from build123d import *

# Parameters (mm, degrees)
SKETCH1_W            = 96
SKETCH1_H            = 11.5
BOSS_EXTRUDE1_DEPTH  = 1
BOSS_EXTRUDE2_DEPTH  = 96
SKETCH3_W            = 100.030166713
SKETCH3_H            = 53.267661774
CUT_EXTRUDE1_DEPTH   = 96
SKETCH4_W            = 73
SKETCH4_H            = 1
BOSS_EXTRUDE3_DEPTH  = 1
SKETCH5_W            = 73
SKETCH5_H            = 1
BOSS_EXTRUDE4_DEPTH  = 5
SKETCH6_W            = 13
SKETCH6_H            = 1
BOSS_EXTRUDE6_DEPTH  = 5
SKETCH7_W            = 13
SKETCH7_H            = 1
BOSS_EXTRUDE7_DEPTH  = 5
BOSS_EXTRUDE8_DEPTH  = 96
SKETCH10_W           = 73
SKETCH10_H           = 6.414213562
BOSS_EXTRUDE9_DEPTH  = 1
BOSS_EXTRUDE10_DEPTH = 1
BOSS_EXTRUDE11_DEPTH = 1
SKETCH13_R           = 45
SKETCH13_R_2         = 40
SKETCH13_R_3         = 32.5
SKETCH13_R_4         = 27.5
SKETCH13_R_5         = 20
SKETCH13_R_6         = 15
CUT_EXTRUDE2_DEPTH   = 10
BOSS_EXTRUDE12_DEPTH = 1
CIRPATTERN1_COUNT    = 4
BOSS_EXTRUDE14_DEPTH = 1
CIRPATTERN2_COUNT    = 4
BOSS_EXTRUDE15_DEPTH = 1
CIRPATTERN3_COUNT    = 4


with BuildPart() as part:
    # Sketch1 → Boss-Extrude1 (new body)
    with BuildSketch(Plane.XY):
        with Locations((48, 5.75)):
            Rectangle(SKETCH1_W, SKETCH1_H)
    extrude(amount=BOSS_EXTRUDE1_DEPTH)

    # Sketch2 → Boss-Extrude2 (add)
    with BuildSketch(Plane.ZY):
        Polygon((1, 0), (-86.974134086, -87.974134086), (-87.681240867, -87.267027305), (0, 0.414213562), align=None)
    extrude(amount=-BOSS_EXTRUDE2_DEPTH)

    # Sketch3 → Cut-Extrude1 (cut)
    with BuildSketch(Plane.ZY):
        with Locations((-50.015083356, -111.133830887)):
            Rectangle(SKETCH3_W, SKETCH3_H)
    extrude(amount=-CUT_EXTRUDE1_DEPTH, mode=Mode.SUBTRACT)

    # Sketch4 → Boss-Extrude3 (add)
    with BuildSketch(Plane(origin=(0, 11.5, 0), x_dir=(1, 0, 0), z_dir=(0, 1, 0))):
        with Locations((48, -0.5)):
            Rectangle(SKETCH4_W, SKETCH4_H)
    extrude(amount=BOSS_EXTRUDE3_DEPTH)

    # Sketch5 → Boss-Extrude4 (add)
    with BuildSketch(Plane(origin=(0, 0, 0), x_dir=(-1, 0, 0), z_dir=(0, 0, -1))):
        with Locations((-48, 12)):
            Rectangle(SKETCH5_W, SKETCH5_H)
    extrude(amount=BOSS_EXTRUDE4_DEPTH)

    # Sketch6 → Boss-Extrude6 (add)
    with BuildSketch(Plane(origin=(0, 0, 0), x_dir=(-1, 0, 0), z_dir=(0, 0, -1))):
        with Locations((-6.5, 11)):
            Rectangle(SKETCH6_W, SKETCH6_H)
    extrude(amount=BOSS_EXTRUDE6_DEPTH)

    # Sketch7 → Boss-Extrude7 (add)
    with BuildSketch(Plane(origin=(0, 0, 0), x_dir=(-1, 0, 0), z_dir=(0, 0, -1))):
        with Locations((-89.5, 11)):
            Rectangle(SKETCH7_W, SKETCH7_H)
    extrude(amount=BOSS_EXTRUDE7_DEPTH)

    # Sketch8 → Boss-Extrude8 (add)
    with BuildSketch(Plane(origin=(96, 0, 0), x_dir=(0, 0, -1), z_dir=(1, 0, 0))):
        Polygon((83.5, -84.5), (89.914213562, -84.5), (89.914213562, -83.5), (82.5, -83.5), align=None)
    extrude(amount=-BOSS_EXTRUDE8_DEPTH)

    # Sketch10 → Boss-Extrude9 (add)
    with BuildSketch(Plane.XZ.offset(84.5)):
        with Locations((48, -86.707106781)):
            Rectangle(SKETCH10_W, SKETCH10_H)
    extrude(amount=BOSS_EXTRUDE9_DEPTH)

    # Sketch11 → Boss-Extrude10 (add)
    with BuildSketch(Plane.ZY):
        Polygon((-5, 10.5), (-5, 6.02081528), (-94.52081528, -83.5), (-83.914213562, -83.5), (0, 0.414213562), (0, 10.5), align=None)
    extrude(amount=-BOSS_EXTRUDE10_DEPTH)

    # Sketch12 → Boss-Extrude11 (add)
    with BuildSketch(Plane(origin=(96, 0, 0), x_dir=(0, 0, -1), z_dir=(1, 0, 0))):
        Polygon((5, 10.5), (0, 10.5), (0, 0.414213562), (83.914213562, -83.5), (94.52081528, -83.5), (5, 6.02081528), align=None)
    extrude(amount=-BOSS_EXTRUDE11_DEPTH)

    # Sketch13 → Cut-Extrude2 (cut)
    # profile 1 of 3: a face of its own
    with BuildSketch(Plane(origin=(0, -0.5, 0.5), x_dir=(1, 0, 0), z_dir=(0, -0.7071067811865486, 0.7071067811865465))):
        with Locations(Location((48, -59.042893219, 0), (0, 0, 270))):
            Circle(SKETCH13_R)
        with Locations(Location((48, -59.042893219, 0), (0, 0, 270))):
            Circle(SKETCH13_R_2, mode=Mode.SUBTRACT)
    # profile 2 of 3: a face of its own
    with BuildSketch(Plane(origin=(0, -0.5, 0.5), x_dir=(1, 0, 0), z_dir=(0, -0.7071067811865486, 0.7071067811865465))):
        with Locations(Location((48, -59.042893219, 0), (0, 0, 270))):
            Circle(SKETCH13_R_3)
        with Locations(Location((48, -59.042893219, 0), (0, 0, 270))):
            Circle(SKETCH13_R_4, mode=Mode.SUBTRACT)
    # profile 3 of 3: a face of its own
    with BuildSketch(Plane(origin=(0, -0.5, 0.5), x_dir=(1, 0, 0), z_dir=(0, -0.7071067811865486, 0.7071067811865465))):
        with Locations(Location((48, -59.042893219, 0), (0, 0, 270))):
            Circle(SKETCH13_R_5)
        with Locations(Location((48, -59.042893219, 0), (0, 0, 270))):
            Circle(SKETCH13_R_6, mode=Mode.SUBTRACT)
    extrude(amount=-CUT_EXTRUDE2_DEPTH, mode=Mode.SUBTRACT)


with BuildPart() as cut_extrude2_piece_1:
    # of the separate pieces the step leaves, piece 1, a body of its own (cut_extrude2_pieces)
    add(part.part.solids().sort_by_distance((0, 11.5, 1))[0])



with BuildPart() as cut_extrude2_piece_2:
    # of the separate pieces the step leaves, piece 2, a body of its own (cut_extrude2_pieces)
    add(part.part.solids().sort_by_distance((48, -70.533901423, -69.533901423))[0])


with BuildPart() as cut_extrude2_piece_3:
    # of the separate pieces the step leaves, piece 3, a body of its own (cut_extrude2_pieces)
    add(part.part.solids().sort_by_distance((48, -61.695066659, -60.695066659))[0])



with BuildPart() as cut_extrude2_piece_4:
    # of the separate pieces the step leaves, piece 4, a body of its own (cut_extrude2_pieces)
    add(part.part.solids().sort_by_distance((48, -52.856231894, -51.856231894))[0])


with BuildPart() as cut_extrude2_piece_1_1:
    add(cut_extrude2_piece_1.part)

    add(cut_extrude2_piece_2.part)  # Boss-Extrude12 merges Cut-Extrude2 piece 2
    # Sketch14 → Boss-Extrude12 (add)
    with BuildSketch(Plane(origin=(0, -0.5, 0.5), x_dir=(1, 0, 0), z_dir=(0, -0.7071067811865486, 0.7071067811865465))):
        with BuildLine():
            Line((45.5, -103.973395108), (45.5, -98.964691775))
            ThreePointArc((45.5, -98.964691775), (48, -99.042893219), (50.5, -98.964691775))
            Line((50.5, -98.964691775), (50.5, -103.973395108))
            ThreePointArc((50.5, -103.973395108), (48, -104.042893219), (45.5, -103.973395108))
        make_face()
    boss_extrude12 = extrude(amount=-BOSS_EXTRUDE12_DEPTH)

    # CirPattern1: Boss-Extrude12 ×4 about axis
    cirpattern1_axis = Axis((48, -41.749630176, -41.749630176), (0, -0.7071067811865476, 0.7071067811865476))
    for i in range(1, CIRPATTERN1_COUNT):
        add(boss_extrude12.rotate(cirpattern1_axis, i * 360 / CIRPATTERN1_COUNT))



with BuildPart() as cut_extrude2_piece_3_1:
    add(cut_extrude2_piece_3.part)

    add(cut_extrude2_piece_4.part)  # Boss-Extrude14 merges Cut-Extrude2 piece 4
    # Sketch16 → Boss-Extrude14 (add)
    with BuildSketch(Plane(origin=(0, -0.5, 0.5), x_dir=(1, 0, 0), z_dir=(0, -0.7071067811865486, 0.7071067811865465))):
        with BuildLine():
            Line((45.5, -73.833092677), (45.5, -78.886028052))
            ThreePointArc((45.5, -78.886028052), (48, -79.042893219), (50.5, -78.886028052))
            Line((50.5, -78.886028052), (50.5, -73.833092677))
            ThreePointArc((50.5, -73.833092677), (48, -74.042893219), (45.5, -73.833092677))
        make_face()
    boss_extrude14 = extrude(amount=-BOSS_EXTRUDE14_DEPTH)

    # CirPattern2: Boss-Extrude14 ×4 about axis
    cirpattern2_axis = Axis((48, -41.749630176, -41.749630176), (0, -0.7071067811865476, 0.7071067811865476))
    for i in range(1, CIRPATTERN2_COUNT):
        add(boss_extrude14.rotate(cirpattern2_axis, i * 360 / CIRPATTERN2_COUNT))


with BuildPart() as cut_extrude2_piece_1_2:
    add(cut_extrude2_piece_1_1.part)

    add(cut_extrude2_piece_3_1.part)  # Boss-Extrude15 merges Cut-Extrude2 piece 3
    # Sketch17 → Boss-Extrude15 (add)
    with BuildSketch(Plane(origin=(0, -0.5, 0.5), x_dir=(1, 0, 0), z_dir=(0, -0.7071067811865486, 0.7071067811865465))):
        with BuildLine():
            Line((25.434059771, -43.325757934), (21.851195056, -39.742893219))
            ThreePointArc((21.851195056, -39.742893219), (23.413288551, -37.788631996), (25.121081398, -35.960322227))
            Line((25.121081398, -35.960322227), (28.656656321, -39.49589715))
            ThreePointArc((28.656656321, -39.49589715), (26.958042443, -41.337356735), (25.434059771, -43.325757934))
        make_face()
    boss_extrude15 = extrude(amount=-BOSS_EXTRUDE15_DEPTH)

    # CirPattern3: Boss-Extrude15 ×4 about axis
    cirpattern3_axis = Axis((48, -41.749630176, -41.749630176), (0, -0.7071067811865487, 0.7071067811865465))
    for i in range(1, CIRPATTERN3_COUNT):
        add(boss_extrude15.rotate(cirpattern3_axis, i * 360 / CIRPATTERN3_COUNT))


solid = cut_extrude2_piece_1_2.part
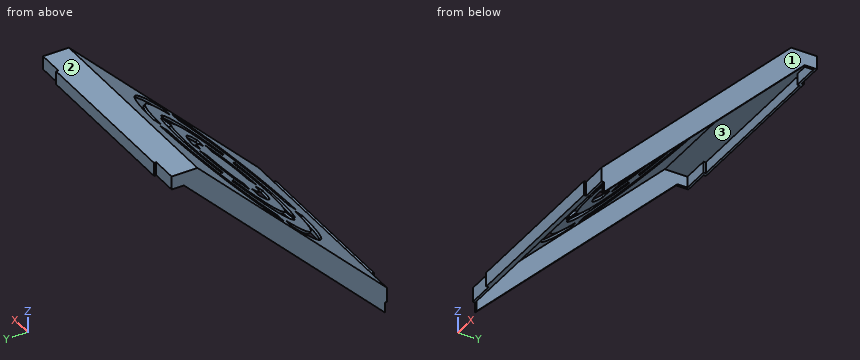
Part model, mm, in its own coordinate system. Face numbers are marked on the shaded views. Give positions to 0.01 mm unless a question says otherwise; leave off trailing zeros. Loops run counter-clockwise (first coordinate to the right, second up) from the corner with the lowest first, then second, coordinate; pieces in that order, holes last. Notation, with made-up numbers: M 22.5,46 L 54.5,46 A29 cw 54.5,69 Z; hole C -40,89 d10. An arc over 180 degrees is marked long. Put each result on its own line as item: value. Start each with the question number.
1) Saw through at C-C (y = -33.5). State how many separate pieces and enclosed holes the cut face has, then the cut area to 3 significant figures.
2) Pull direction X, two halves, no side cores. Call the marked faces 1, 2 and 3: +X half, -X half, draft (parallel to the pull), parting line (faces both ways), or undercut.
3) Saw through at A-A (x = 90.5). List the corners of the cut face in (y, z), then the cut area to 3 significant figures.
4) Saw through at B-B (x = 18). List the corners of the cut face in (y, z), then the cut area to 3 significant figures.
5) Flat gauge pins, fed straight in: pin 1 (5 mm diameter, centred on x = 91.5, z = -87.5, fed in from -Y); pin 2 (0.5 mm diameter, centred on y = -85, z = -85.5, fed in from -X); pin 3 (12 mm diameter, centred on x = 74, y = -49.5, fed in from -Z). Where does each tip first touch, or does it go through?
6) Probe probe 1 along Y at (x, z) = (39.5, -4); probe 2 along Y at (x, z) = (14.5, -3.5); probe 3 along Z at (x, y) = (27, 8). List the from-to ranges inside material, lowest first.
Numbers:
1. separate pieces: 7
1. enclosed holes: 0
1. area: 107 mm^2
2. face 1: +X half
2. face 2: draft
2. face 3: undercut
3. outline: M -84.5,-89.91 L -83.5,-89.91 L -83.5,-83.91 L -52,-52.41 L -52.71,-51.71 L -84.5,-83.5 Z; M -44.02,-43.02 L -43.31,-43.72 L -39.77,-40.19 L -40.48,-39.48 Z; M -31.79,-30.79 L -31.08,-31.5 L 0.41,0 L 10.5,0 L 10.5,-5 L 11.5,-5 L 11.5,1 L 0,1 Z
3. area: 117 mm^2
4. outline: M -85.5,-89.91 L -83.5,-89.91 L -83.5,-83.91 L -65.26,-65.67 L -65.97,-64.97 L -84.5,-83.5 L -85.5,-83.5 Z; M -60.96,-59.96 L -60.25,-60.67 L -50.38,-50.8 L -51.09,-50.09 Z; M -33.41,-32.41 L -32.7,-33.12 L -22.83,-23.25 L -23.54,-22.54 Z; M -18.53,-17.53 L -17.83,-18.24 L 0.41,0 L 11.5,0 L 11.5,-5 L 12.5,-5 L 12.5,1 L 0,1 Z
4. area: 110 mm^2
5. pin 1: y = -84.5
5. pin 2: x = 11.5
5. pin 3: z = -55.91
6. probe 1: -5 to -3.59, 11.5 to 12.5
6. probe 2: -4.5 to -3.09, 11.5 to 12.5
6. probe 3: 0 to 1
